```python
from build123d import *

# Parameters (mm, degrees)
EXTRUDE_1_DEPTH         = 3
SKETCH_3_W              = 11
SKETCH_3_H              = 7.5
SKETCH_3_H_2            = 11
SKETCH_3_H_3            = 15
EXTRUDE_3_DEPTH         = 20
HOLE_WIZARD_M3_1_REACH  = 211.762
HOLE_WIZARD_M3_1_BORE_R = 1.7
FILLET_1_R              = 10


with BuildPart() as part:
    # Sketch 1 → Extrude 1 (new body)
    with BuildSketch(Plane(origin=(0, 0, 0), x_dir=(1, 0, 0), z_dir=(0, 1, 0))):
        Polygon((-100, 60), (-70, 60), (-70, 20), (70, 20), (70, 60), (100, 60), (100, -60), (70, -60), (70, -20), (-70, -20), (-70, -60), (-100, -60), align=None)
    extrude(amount=EXTRUDE_1_DEPTH)

    # Sketch 3 → Extrude 3 (add)
    with BuildSketch(Plane.XZ):
        with Locations((-94.5, -3.75)):
            Rectangle(SKETCH_3_W, SKETCH_3_H)
        with Locations((-94.5, 3.75)):
            Rectangle(SKETCH_3_W, SKETCH_3_H)
        with Locations((-94.5, 54.5)):
            Rectangle(SKETCH_3_W, SKETCH_3_H_2)
        with Locations((-94.5, -54.5)):
            Rectangle(SKETCH_3_W, SKETCH_3_H_2)
        with Locations((-75.5, 54.5)):
            Rectangle(SKETCH_3_W, SKETCH_3_H_2)
        with Locations((-75.5, -54.5)):
            Rectangle(SKETCH_3_W, SKETCH_3_H_2)
        with Locations((-75.5, 0)):
            Rectangle(SKETCH_3_W, SKETCH_3_H_3)
    extrude(amount=EXTRUDE_3_DEPTH)

    # Hole Wizard M3 _ _1 bore → Hole Wizard M3 _ _1 (cut, up to next)
    with BuildSketch(Plane.ZY.offset(100), mode=Mode.PRIVATE) as hole_wizard_m3_1_sk1:
        with Locations((-3, -5.5)):
            Circle(HOLE_WIZARD_M3_1_BORE_R)
    hole_wizard_m3_1_tool1 = extrude(hole_wizard_m3_1_sk1.sketch, amount=-HOLE_WIZARD_M3_1_REACH, mode=Mode.PRIVATE) & part.part
    # Hole Wizard M3 _ _1 bore → Hole Wizard M3 _ _1 (cut, up to next)
    with BuildSketch(Plane.ZY.offset(100), mode=Mode.PRIVATE) as hole_wizard_m3_1_sk2:
        with Locations((-3, -14.5)):
            Circle(HOLE_WIZARD_M3_1_BORE_R)
    hole_wizard_m3_1_tool2 = extrude(hole_wizard_m3_1_sk2.sketch, amount=-HOLE_WIZARD_M3_1_REACH, mode=Mode.PRIVATE) & part.part
    # Hole Wizard M3 _ _1 bore → Hole Wizard M3 _ _1 (cut, up to next)
    with BuildSketch(Plane.ZY.offset(100), mode=Mode.PRIVATE) as hole_wizard_m3_1_sk3:
        with Locations((-53.3, -5.5)):
            Circle(HOLE_WIZARD_M3_1_BORE_R)
    hole_wizard_m3_1_tool3 = extrude(hole_wizard_m3_1_sk3.sketch, amount=-HOLE_WIZARD_M3_1_REACH, mode=Mode.PRIVATE) & part.part
    # Hole Wizard M3 _ _1 bore → Hole Wizard M3 _ _1 (cut, up to next)
    with BuildSketch(Plane.ZY.offset(100), mode=Mode.PRIVATE) as hole_wizard_m3_1_sk4:
        with Locations((-53.3, -14.5)):
            Circle(HOLE_WIZARD_M3_1_BORE_R)
    hole_wizard_m3_1_tool4 = extrude(hole_wizard_m3_1_sk4.sketch, amount=-HOLE_WIZARD_M3_1_REACH, mode=Mode.PRIVATE) & part.part
    # Hole Wizard M3 _ _1 bore → Hole Wizard M3 _ _1 (cut, up to next)
    with BuildSketch(Plane.ZY.offset(100), mode=Mode.PRIVATE) as hole_wizard_m3_1_sk5:
        with Locations((53.3, -5.5)):
            Circle(HOLE_WIZARD_M3_1_BORE_R)
    hole_wizard_m3_1_tool5 = extrude(hole_wizard_m3_1_sk5.sketch, amount=-HOLE_WIZARD_M3_1_REACH, mode=Mode.PRIVATE) & part.part
    # Hole Wizard M3 _ _1 bore → Hole Wizard M3 _ _1 (cut, up to next)
    with BuildSketch(Plane.ZY.offset(100), mode=Mode.PRIVATE) as hole_wizard_m3_1_sk6:
        with Locations((53.3, -14.5)):
            Circle(HOLE_WIZARD_M3_1_BORE_R)
    hole_wizard_m3_1_tool6 = extrude(hole_wizard_m3_1_sk6.sketch, amount=-HOLE_WIZARD_M3_1_REACH, mode=Mode.PRIVATE) & part.part
    # Hole Wizard M3 _ _1 bore → Hole Wizard M3 _ _1 (cut, up to next)
    with BuildSketch(Plane.ZY.offset(100), mode=Mode.PRIVATE) as hole_wizard_m3_1_sk7:
        with Locations((3, -14.5)):
            Circle(HOLE_WIZARD_M3_1_BORE_R)
    hole_wizard_m3_1_tool7 = extrude(hole_wizard_m3_1_sk7.sketch, amount=-HOLE_WIZARD_M3_1_REACH, mode=Mode.PRIVATE) & part.part
    # Hole Wizard M3 _ _1 bore → Hole Wizard M3 _ _1 (cut, up to next)
    with BuildSketch(Plane.ZY.offset(100), mode=Mode.PRIVATE) as hole_wizard_m3_1_sk8:
        with Locations((3, -5.5)):
            Circle(HOLE_WIZARD_M3_1_BORE_R)
    hole_wizard_m3_1_tool8 = extrude(hole_wizard_m3_1_sk8.sketch, amount=-HOLE_WIZARD_M3_1_REACH, mode=Mode.PRIVATE) & part.part
    hole_wizard_m3_1_1 = hole_wizard_m3_1_tool1.solids().sort_by_distance((-100, -5.5, -3))[0]
    add(hole_wizard_m3_1_1, mode=Mode.SUBTRACT)
    hole_wizard_m3_1_2 = hole_wizard_m3_1_tool2.solids().sort_by_distance((-100, -14.5, -3))[0]
    add(hole_wizard_m3_1_2, mode=Mode.SUBTRACT)
    hole_wizard_m3_1_3 = hole_wizard_m3_1_tool3.solids().sort_by_distance((-100, -5.5, -53.3))[0]
    add(hole_wizard_m3_1_3, mode=Mode.SUBTRACT)
    hole_wizard_m3_1_4 = hole_wizard_m3_1_tool4.solids().sort_by_distance((-100, -14.5, -53.3))[0]
    add(hole_wizard_m3_1_4, mode=Mode.SUBTRACT)
    hole_wizard_m3_1_5 = hole_wizard_m3_1_tool5.solids().sort_by_distance((-100, -5.5, 53.3))[0]
    add(hole_wizard_m3_1_5, mode=Mode.SUBTRACT)
    hole_wizard_m3_1_6 = hole_wizard_m3_1_tool6.solids().sort_by_distance((-100, -14.5, 53.3))[0]
    add(hole_wizard_m3_1_6, mode=Mode.SUBTRACT)
    hole_wizard_m3_1_7 = hole_wizard_m3_1_tool7.solids().sort_by_distance((-100, -14.5, 3))[0]
    add(hole_wizard_m3_1_7, mode=Mode.SUBTRACT)
    hole_wizard_m3_1_8 = hole_wizard_m3_1_tool8.solids().sort_by_distance((-100, -5.5, 3))[0]
    add(hole_wizard_m3_1_8, mode=Mode.SUBTRACT)
    hole_wizard_m3_1 = hole_wizard_m3_1_1 + hole_wizard_m3_1_2 + hole_wizard_m3_1_3 + hole_wizard_m3_1_4 + hole_wizard_m3_1_5 + hole_wizard_m3_1_6 + hole_wizard_m3_1_7 + hole_wizard_m3_1_8  # Hole Wizard M3 _ _1 as one shape, for the pattern or mirror that repeats it

    # Mirror 1: Hole Wizard M3 _ _1 mirrored; each copy of Hole Wizard M3 _ _1 runs up to whatever stops it at its own place
    mirror_1_before = part.part  # the part as the pattern finds it: every copy runs up to it
    mirror_1_hole_wizard_m3_1_long1 = extrude(hole_wizard_m3_1_sk1.sketch, amount=-HOLE_WIZARD_M3_1_REACH, mode=Mode.PRIVATE)
    mirror_1_hole_wizard_m3_1_long2 = extrude(hole_wizard_m3_1_sk2.sketch, amount=-HOLE_WIZARD_M3_1_REACH, mode=Mode.PRIVATE)
    mirror_1_hole_wizard_m3_1_long3 = extrude(hole_wizard_m3_1_sk3.sketch, amount=-HOLE_WIZARD_M3_1_REACH, mode=Mode.PRIVATE)
    mirror_1_hole_wizard_m3_1_long4 = extrude(hole_wizard_m3_1_sk4.sketch, amount=-HOLE_WIZARD_M3_1_REACH, mode=Mode.PRIVATE)
    mirror_1_hole_wizard_m3_1_long5 = extrude(hole_wizard_m3_1_sk5.sketch, amount=-HOLE_WIZARD_M3_1_REACH, mode=Mode.PRIVATE)
    mirror_1_hole_wizard_m3_1_long6 = extrude(hole_wizard_m3_1_sk6.sketch, amount=-HOLE_WIZARD_M3_1_REACH, mode=Mode.PRIVATE)
    mirror_1_hole_wizard_m3_1_long7 = extrude(hole_wizard_m3_1_sk7.sketch, amount=-HOLE_WIZARD_M3_1_REACH, mode=Mode.PRIVATE)
    mirror_1_hole_wizard_m3_1_long8 = extrude(hole_wizard_m3_1_sk8.sketch, amount=-HOLE_WIZARD_M3_1_REACH, mode=Mode.PRIVATE)
    mirror_1_hole_wizard_m3_1_tool1_1 = mirror_1_hole_wizard_m3_1_long1.mirror(Plane(origin=(0, 0, 0), x_dir=(0, 0, 1), z_dir=(1, 0, 0))) & mirror_1_before
    add(mirror_1_hole_wizard_m3_1_tool1_1.solids().sort_by_distance((100, -5.5, -3))[0], mode=Mode.SUBTRACT)
    mirror_1_hole_wizard_m3_1_tool2_1 = mirror_1_hole_wizard_m3_1_long2.mirror(Plane(origin=(0, 0, 0), x_dir=(0, 0, 1), z_dir=(1, 0, 0))) & mirror_1_before
    add(mirror_1_hole_wizard_m3_1_tool2_1.solids().sort_by_distance((100, -14.5, -3))[0], mode=Mode.SUBTRACT)
    mirror_1_hole_wizard_m3_1_tool3_1 = mirror_1_hole_wizard_m3_1_long3.mirror(Plane(origin=(0, 0, 0), x_dir=(0, 0, 1), z_dir=(1, 0, 0))) & mirror_1_before
    add(mirror_1_hole_wizard_m3_1_tool3_1.solids().sort_by_distance((100, -5.5, -53.3))[0], mode=Mode.SUBTRACT)
    mirror_1_hole_wizard_m3_1_tool4_1 = mirror_1_hole_wizard_m3_1_long4.mirror(Plane(origin=(0, 0, 0), x_dir=(0, 0, 1), z_dir=(1, 0, 0))) & mirror_1_before
    add(mirror_1_hole_wizard_m3_1_tool4_1.solids().sort_by_distance((100, -14.5, -53.3))[0], mode=Mode.SUBTRACT)
    mirror_1_hole_wizard_m3_1_tool5_1 = mirror_1_hole_wizard_m3_1_long5.mirror(Plane(origin=(0, 0, 0), x_dir=(0, 0, 1), z_dir=(1, 0, 0))) & mirror_1_before
    add(mirror_1_hole_wizard_m3_1_tool5_1.solids().sort_by_distance((100, -5.5, 53.3))[0], mode=Mode.SUBTRACT)
    mirror_1_hole_wizard_m3_1_tool6_1 = mirror_1_hole_wizard_m3_1_long6.mirror(Plane(origin=(0, 0, 0), x_dir=(0, 0, 1), z_dir=(1, 0, 0))) & mirror_1_before
    add(mirror_1_hole_wizard_m3_1_tool6_1.solids().sort_by_distance((100, -14.5, 53.3))[0], mode=Mode.SUBTRACT)
    mirror_1_hole_wizard_m3_1_tool7_1 = mirror_1_hole_wizard_m3_1_long7.mirror(Plane(origin=(0, 0, 0), x_dir=(0, 0, 1), z_dir=(1, 0, 0))) & mirror_1_before
    add(mirror_1_hole_wizard_m3_1_tool7_1.solids().sort_by_distance((100, -14.5, 3))[0], mode=Mode.SUBTRACT)
    mirror_1_hole_wizard_m3_1_tool8_1 = mirror_1_hole_wizard_m3_1_long8.mirror(Plane(origin=(0, 0, 0), x_dir=(0, 0, 1), z_dir=(1, 0, 0))) & mirror_1_before
    add(mirror_1_hole_wizard_m3_1_tool8_1.solids().sort_by_distance((100, -5.5, 3))[0], mode=Mode.SUBTRACT)

    # Fillet 1
    # the kernel refuses this fillet: 10 mm, written as the material it takes off along each edge
    with BuildSketch(Plane(origin=(-81, 0, 60), x_dir=(0, 0, -1), z_dir=(-1, 0, 0))) as fillet_1_piece_1:
        with BuildLine():
            CenterArc((FILLET_1_R, -FILLET_1_R), FILLET_1_R, 90, 90)
            Line((0, -FILLET_1_R), (0, 0))
            Line((0, 0), (FILLET_1_R, 0))
        make_face()
    extrude(amount=8, mode=Mode.SUBTRACT)
    with BuildSketch(Plane(origin=(-64, -20, 60), x_dir=(0, 1, 0), z_dir=(-1, 0, 0)), Plane(origin=(-125, -20, -60), x_dir=(0, 1, 0), z_dir=(1, 0, 0)), Plane(origin=(-106, -20, -60), x_dir=(0, 1, 0), z_dir=(1, 0, 0))) as fillet_1_piece_2:
        with BuildLine():
            CenterArc((FILLET_1_R, FILLET_1_R), FILLET_1_R, 180, 90)
            Line((0, FILLET_1_R), (0, 0))
            Line((0, 0), (FILLET_1_R, 0))
        make_face()
    extrude(amount=61, mode=Mode.SUBTRACT)
    with BuildSketch(Plane(origin=(-106, -20, 60), x_dir=(0, 1, 0), z_dir=(1, 0, 0))) as fillet_1_piece_3:
        with BuildLine():
            CenterArc((FILLET_1_R, -FILLET_1_R), FILLET_1_R, 90, 90)
            Line((0, -FILLET_1_R), (0, 0))
            Line((0, 0), (FILLET_1_R, 0))
        make_face()
    extrude(amount=61, mode=Mode.SUBTRACT)
    with BuildSketch(Plane(origin=(-89, 0, -60), x_dir=(0, 1, 0), z_dir=(1, 0, 0))) as fillet_1_piece_4:
        with BuildLine():
            CenterArc((FILLET_1_R, FILLET_1_R), FILLET_1_R, 180, 90)
            Line((0, FILLET_1_R), (0, 0))
            Line((0, 0), (FILLET_1_R, 0))
        make_face()
    extrude(amount=8, mode=Mode.SUBTRACT)


solid = part.part
```
For this review, take the finished solid that the model builds, in its own axes (mm). A direction names the side the tool comes from. Give positions to 0.01 mm unless a question says otherwise; leave off trailing zeros. Loops run counter-clockwise (first coordinate to the right, second up) from the corner with the lowest first, then second, coordinate; pieces in that order, holes last. Notation, with made-up numbers: M 4.5,3.25 L 19.5,3.25 A18 cw 19.5,19.25 Z; hole C 21.25,-15.5 d8. An arc over 180 degrees is marked long. One line per item, written item: value. Start each with the question number.
Q1. For L1, parallel to Y at x = -96, z = -3; L2, parallel to X at y = -0.75, z = -52.5; L3, parallel to Y at x = -76.75, z = 53.3, list the stretches that pass through material, from the lowest coordinate up.
Q2. Add section B-B (x = -72.5). Count the separate pieces of the cut face and the enclosed holes in it, and give its area (3 significant figures).
Q3. Add section A-A (z = -29). Give the boundary of the cut face in (x, y).
Q4. Draft analysis for pull direction X (two halves, no side actions). For faces 1 (the face through (-100, -6, -5)), 2 (the face through (-84.94, 0.76, 53.82)), 3 (the face through (-75.42, -17.15, 56.99)), state which applies: released by +X, released by -X, zero draft, split by the parting line, or undercut.
Q5. Machinability: for faces 4 (the face through (-95, -3, 60)), 5 (the face through (-76, -10, 49)), which of the approach directions +Z, -Z, +X, -X, +Y, -Y give a long, thin tool a straight path to every point of the face, cutting with its end or side? Answer none if there is none.
Q6. Add section C-C (x = 14). Give the boundary of the cut face in (y, z), and give its area (3 significant figures).
Q7. Clearance check with flat-ended pins moving along their axes: pin 1 Ø12 at (x, z) = (42.5, -11) entering from -Y; pin 2 Ø4 at (y, z) = (-5.5, -53.3) entering from +X; pin 3 Ø3.5 at (x, y) = (-75.5, -12.5) entering from -Z. State where each tip first meets the part, or that it passes through.
Reply:
1. L1: -20 to -16.2, -12.8 to -7.2, -3.8 to 3
1. L2: -100 to -89, -81 to -70
1. L3: -19.44 to -16.2, -12.8 to -7.2, -3.8 to 3
2. separate pieces: 1
2. enclosed holes: 8
2. area: 984 mm²
3. outline: M -100,0 L -70,0 L -70,3 L -100,3 Z; M 70,0 L 100,0 L 100,3 L 70,3 Z
4. face 1: released by -X
4. face 2: undercut
4. face 3: zero draft
5. face 4: +Z, +X, -X, +Y, -Y
5. face 5: +X, -X, -Y
6. outline: M 0,-20 L 3,-20 L 3,20 L 0,20 Z
6. area: 120 mm²
7. pin 1: y = 0
7. pin 2: x = -70
7. pin 3: z = -59.97
